Read the model definition and answer for the solid it produces. Units are mm, in the model's axes. Face numbers are marked on the shaded views. Give positions to 0.01 mm unless a question says otherwise; leave off trailing zeros. Order: outer loops, then holes, each group sorted by start corner. A loop starts at its lowest first (then second) coordinate and runs counter-clockwise, first axis right, second up. Notation, with made-up numbers: M 25.5,26.5 L 52.5,26.5 A20 cw 52.5,55.5 Z; hole C 50,48 d10. An arc over 180 degrees is marked long. One line per item, written item: value.
from build123d import *

# Parameters (mm, degrees)
SKETCH1_W           = 76.2
SKETCH1_H           = 102.603301604
SKETCH1_R           = 2.6035
BOSS_EXTRUDE1_DEPTH = 9.525
SKETCH2_R           = 2.6035
CUT_EXTRUDE1_DEPTH  = 122.484770136


with BuildPart() as part:
    # Sketch1 → Boss-Extrude1 (new body)
    with BuildSketch(Plane(origin=(0, 69.975, 0), x_dir=(1, 0, 0), z_dir=(0, 1, 0))):
        Rectangle(SKETCH1_W, SKETCH1_H)
        with Locations(Location((25.4, -25.4, 0), (0, 0, 90))):
            Circle(SKETCH1_R, mode=Mode.SUBTRACT)
        with Locations(Location((-25.4, -25.4, 0), (0, 0, 90))):
            Circle(SKETCH1_R, mode=Mode.SUBTRACT)
        with Locations(Location((-25.4, 25.4, 0), (0, 0, 90))):
            Circle(SKETCH1_R, mode=Mode.SUBTRACT)
        with Locations(Location((25.4, 25.4, 0), (0, 0, 90))):
            Circle(SKETCH1_R, mode=Mode.SUBTRACT)
    extrude(amount=BOSS_EXTRUDE1_DEPTH)

    # Sketch2 → Cut-Extrude1 (cut, through all)
    with BuildSketch(Plane.ZY.offset(38.1)):
        with Locations((0, 74.7375)):
            Circle(SKETCH2_R)
        with Locations((-38.476238101, 74.7375)):
            Circle(SKETCH2_R)
        with Locations((38.476238101, 74.7375)):
            Circle(SKETCH2_R)
    extrude(amount=-CUT_EXTRUDE1_DEPTH, mode=Mode.SUBTRACT)


solid = part.part
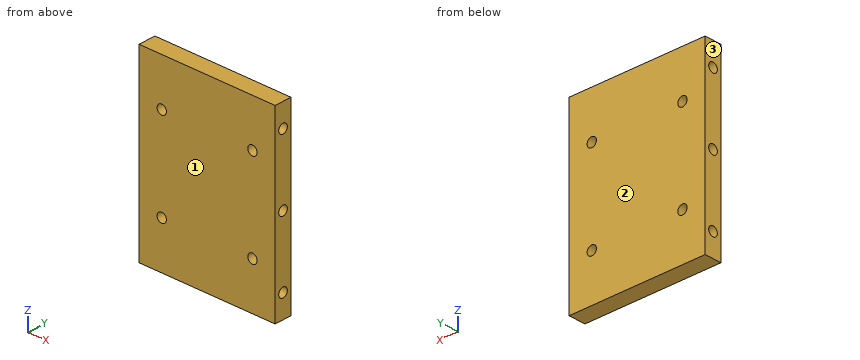
1) Determine the mould class of the marked faces 1, 2 and 3 for opening direction Y: +Y half, -Y half, draft (parallel to the pull), parting line (faces both ways), or undercut.
Reported:
face 1: -Y half
face 2: +Y half
face 3: draft
2) Find section B-B, the plane x = -25.4. Write down the section's boundary in (y, z) (1 decimal), plus the area to 3 significant figures.
Reported:
outline: M 70,-51.3 L 79.5,-51.3 L 79.5,-28 L 70,-28 Z; M 70,-22.8 L 79.5,-22.8 L 79.5,22.8 L 70,22.8 Z; M 70,28 L 79.5,28 L 79.5,51.3 L 70,51.3 Z; hole C 74.7,-38.5 d5.2; hole C 74.7,0 d5.2; hole C 74.7,38.5 d5.2
area: 814 mm^2
3) Find section A-A, the plane z = 0. Write down the section's boundary in (x, y) (3 decimals).
Reported:
outline: M -38.1,69.975 L 38.1,69.975 L 38.1,72.134 L -38.1,72.134 Z; M -38.1,77.341 L 38.1,77.341 L 38.1,79.5 L -38.1,79.5 Z
4) Find section D-D, the plane x = 13. Write down the section's boundary in (y, z) (1 decimal), plus the area to 3 significant figures.
Reported:
outline: M 70,-51.3 L 79.5,-51.3 L 79.5,51.3 L 70,51.3 Z; hole C 74.7,-38.5 d5.2; hole C 74.7,0 d5.2; hole C 74.7,38.5 d5.2
area: 913 mm^2
5) Consider probe 1 along X at (y, z) = (76, -25.4); probe 2 along Z at (x, y) = (29.5, 75.5); probe 3 along Z at (x, y) = (-20, 72.5). Determine where each line is inside the solid, lowest interval first.
Reported:
probe 1: x = -38.1 to -28, -22.8 to 22.8, 28 to 38.1
probe 2: z = -51.3 to -40.97, -35.99 to -2.49, 2.49 to 35.99, 40.97 to 51.3
probe 3: z = -51.3 to -39.81, -37.15 to -1.33, 1.33 to 37.15, 39.81 to 51.3
6) This flat-tipped pin is pushed along its axis until it touches: pin 1 Ø3 at (y, z) = (74.74, -38.48) entering from -X. Where does it stop, or does it pass through?
Reported:
pin 1: passes through
7) Find section C-C, the plane z = 25.4. Write down the section's boundary in (x, y) (1 decimal).
Reported:
outline: M -38.1,70 L -28,70 L -28,79.5 L -38.1,79.5 Z; M -22.8,70 L 22.8,70 L 22.8,79.5 L -22.8,79.5 Z; M 28,70 L 38.1,70 L 38.1,79.5 L 28,79.5 Z
